Here's how the part is built. I have some questions about the finished solid (model axes, mm). Round coordinates to 2 decimals unless told otherwise and drop trailing zeros. Loops run counter-clockwise (first coordinate to the right, second up) from the corner with the lowest first, then second, coordinate; pieces in that order, holes last. Notation, with made-up numbers: M -39.5,-10 L -34.5,-10 A23 cw -34.5,20 Z; hole C 13,81.5 d8. An arc over 180 degrees is marked long. Answer as a JSON object with one key per item and string values.
from build123d import *

# Parameters (mm, degrees)
SKETCH2_W           = 50.8
SKETCH2_H           = 105.799998966
SKETCH2_R           = 14.2875
SKETCH2_R_2         = 2.38125
BOSS_EXTRUDE1_DEPTH = 6.35
SKETCH6_R           = 2.0828
CUT_EXTRUDE1_DEPTH  = 51.8


with BuildPart() as part:
    # Sketch2 → Boss-Extrude1 (new body)
    with BuildSketch(Plane.XY):
        with Locations((0, -27.499999483)):
            Rectangle(SKETCH2_W, SKETCH2_H)
        Circle(SKETCH2_R, mode=Mode.SUBTRACT)
        with Locations((0, -54.999998966)):
            Circle(SKETCH2_R, mode=Mode.SUBTRACT)
        with Locations((-17.960512242, -17.960512242)):
            Circle(SKETCH2_R_2, mode=Mode.SUBTRACT)
        with Locations((17.960512242, 17.960512242)):
            Circle(SKETCH2_R_2, mode=Mode.SUBTRACT)
    extrude(amount=BOSS_EXTRUDE1_DEPTH)

    # Sketch6 → Cut-Extrude1 (cut, through all)
    with BuildSketch(Plane(origin=(25.4, 0, 0), x_dir=(0, 0, -1), z_dir=(1, 0, 0))):
        with Locations((-3.175, -65.159998966)):
            Circle(SKETCH6_R)
        with Locations((-3.175, -46.109998966)):
            Circle(SKETCH6_R)
    extrude(amount=-CUT_EXTRUDE1_DEPTH, mode=Mode.SUBTRACT)


solid = part.part
Item 1: For P1, Ø4.5, axis at x = -17.96, y = -17.96, coming from the -Z side, with a flat end and sliding along its axis, tell me the tip position at first contact or that it passes through.
Solution:
{"P1": "passes through"}
Item 2: We'd pull the mould along Z, two halves only. Please class faces 1 (the face through (0, -27, 0)), 2 (the face through (-18.967, -44.045, 3.446)), 3 (the face through (25.4, -28, 3)): +Z half, -Z half, draft (parallel to the pull), parting line (faces both ways), or undercut.
Solution:
{"face 1": "-Z half", "face 2": "undercut", "face 3": "draft"}
Item 3: I want a section at D-D on y = -45. List the corners of the cut face in (x, z) for me.
Solution:
{"outline": "M -25.4,0 L -10.2,0 L -10.2,1.41 L -25.4,1.41 Z; M -25.4,4.94 L -10.2,4.94 L -10.2,6.35 L -25.4,6.35 Z; M 10.2,0 L 25.4,0 L 25.4,1.41 L 10.2,1.41 Z; M 10.2,4.94 L 25.4,4.94 L 25.4,6.35 L 10.2,6.35 Z"}
Item 4: I want a section at C-C on y = 0. List the corners of the cut face in (x, z) for me, plus the area to 3 significant figures.
Solution:
{"outline": "M -25.4,0 L -14.29,0 L -14.29,6.35 L -25.4,6.35 Z; M 14.29,0 L 25.4,0 L 25.4,6.35 L 14.29,6.35 Z", "area": "141 mm2"}
Item 5: I want a section at B-B on z = 3.5. List the corners of the cut face in (x, y) for me (1 decimal).
Solution:
{"outline": "M -25.4,-80.4 L 25.4,-80.4 L 25.4,-67.2 L 7.4,-67.2 A14.3 cw -7.4,-67.2 L -25.4,-67.2 Z; M -25.4,-63.1 L -11.8,-63.1 A14.3 cw -12.5,-48.2 L -25.4,-48.2 Z; M -25.4,-44.1 L -9.2,-44.1 A14.3 cw 9.2,-44.1 L 25.4,-44.1 L 25.4,25.4 L -25.4,25.4 Z; M 11.8,-63.1 L 25.4,-63.1 L 25.4,-48.2 L 12.5,-48.2 A14.3 cw Z; hole C -18,-18 d4.8; hole C 0,0 d28.6; hole C 18,18 d4.8"}
Item 6: I want a section at A-A on x = 0. List the corners of the cut face in (y, z) for me, plus the area to 3 significant figures.
Solution:
{"outline": "M -80.4,0 L -69.29,0 L -69.29,6.35 L -80.4,6.35 Z; M -40.71,0 L -14.29,0 L -14.29,6.35 L -40.71,6.35 Z; M 14.29,0 L 25.4,0 L 25.4,6.35 L 14.29,6.35 Z", "area": "309 mm2"}
Item 7: If I drill on L1, parallel to Y at x = 0, z = 1.75; L2, parallel to Y at x = 8, z = 3.25; L3, parallel to Y at x = 16, z = 1.5, over which ranges is the centre line in solid material (lowest first)? Write a range as from..to.
Solution:
{"L1": "y = -80.4..-69.29, -40.71..-14.29, 14.29..25.4", "L2": "y = -80.4..-67.24, -43.16..-11.84, 11.84..25.4", "L3": "y = -80.4..-66.4, -63.92..-47.35, -44.87..16.61, 19.31..25.4"}
